```python
from build123d import *

# Parameters (mm, degrees)
F0_W     = 240
F0_H     = 170
F1_DEPTH = 6
F2_R     = 15
F3_R     = 5


with BuildPart() as f1:
    # F0 (on Top) → F1 (new body)
    with BuildSketch(Plane.XY):
        Rectangle(F0_W, F0_H)
    extrude(amount=F1_DEPTH)

    # F2
    f2_edges = [f1.edges().sort_by_distance(p)[0] for p in [
        (-120, -85, 3),
        (-120, 85, 3),
        (120, 85, 3),
        (120, -85, 3),
    ]]
    fillet(f2_edges, radius=F2_R)

    # F3
    f3_edges = [f1.edges().sort_by_distance(p)[0] for p in [
        (120, 0, 0),
        (115.606602, -80.606602, 0),
        (115.606602, 80.606602, 0),
        (0, -85, 0),
        (0, 85, 0),
        (-115.606602, -80.606602, 0),
        (-115.606602, 80.606602, 0),
        (-120, 0, 0),
    ]]
    fillet(f3_edges, radius=F3_R)


solid = f1.part
```
Design review of the part built by this model. Coordinates are the model's own, in mm. Coordinates: 2 decimals unless noted, no trailing zeros. Write each loop counter-clockwise with the first axis right and the second up, starting at its lowest first coordinate (ties: lowest second). Pieces come first, ordered by that corner, then holes. Notation, with made-up numbers: M 71,33 L 107,33 A7 cw 107,42 Z; hole C 60,87.5 d11. An arc over 180 degrees is marked long. Answer as a JSON object with one key per item and string values.
Item 1: Add section A-A, the plane z = 2.75. Give the boundary of the cut face in (x, y), and give its area (3 significant figures).
Outcome:
{"outline": "M -119.47,-70 A14.47 ccw -105,-84.47 L 105,-84.47 A14.47 ccw 119.47,-70 L 119.47,70 A14.47 ccw 105,84.47 L -105,84.47 A14.47 ccw -119.47,70 Z", "area": "40,200 mm²"}
Item 2: Wall thickness on probe 1 along Y at (x, z) = (86.5, 4.75); probe 2 along X at (y, z) = (-32, 4.75); probe 3 along Y at (x, z) = (-73, 1): over which ranges is each line inside the solid? List them lowest first.
Outcome:
{"probe 1": "-84.99 to 84.99", "probe 2": "-119.99 to 119.99", "probe 3": "-83 to 83"}
Item 3: Insertion check: pin 1 Ø2 at (y, z) = (29.5, 3.5) entering from +X; pin 2 Ø1.5 at (x, z) = (69, 2.5) entering from -Y; pin 3 Ø2 at (x, z) = (17.5, 1) entering from +Y. Each pin has a flat end and moves straight along its axis. Give the tip position at first contact, or say it passes through.
Outcome:
{"pin 1": "x = 119.97", "pin 2": "y = -84.68", "pin 3": "y = 84"}
